For this review, take the finished solid that the model builds, in its own axes (mm). A direction names the side the tool comes from. Give positions to 0.01 mm unless a question says otherwise; leave off trailing zeros. Loops run counter-clockwise (first coordinate to the right, second up) from the corner with the lowest first, then second, coordinate; pieces in that order, holes last. Notation, with made-up numbers: (30.5, 56.5) -> (75.5, 56.5) arc R18 cw to (75.5, 73.5) -> close; hole circle Ø7 at (36, -4.5). An arc over 180 degrees is marked (long way). Answer as CSV lines item,"result". Start each with the question number.
Item 1: Add section A-A on z = -1. State the section outline as (x, y) points, plus the area to 3 significant figures.
Item 2: Clearance check with flat-ended pins moving along their axes: P1, Ø1.5, axis at y = -41.5, z = -13.5, coming from the +X side; P2, Ø5, axis at x = 1, y = -51, coming from the -Z side; P3, Ø2, axis at x = 6, y = -49.5, coming from the +Z side. State where each tip first meets the part, or that it passes through.
Item 3: Add section D-D on x = 6. State the section outline as (y, z) points, plus the area to 3 significant figures.
Item 4: Machinability: for faces 4 (the face through (5, -46, -7.498)), 5 (the face through (5.009, -45.969, -37.974)), which of the approach directions +Z, -Z, +X, -X, +Y, -Y give a long, thin tool a straight path to every point of the face, cutting with its end or side? Answer none if there is none.
Item 5: Add section B-B on y = -44. State the section outline as (x, z) points, plus the area to 3 significant figures.
Item 6: For L1, parallel to Y at x = 7.25, z = 2.5; L2, parallel to Z at x = 6.25, y = -53; L3, parallel to Z at x = 5, y = -50, list the stretches that pass through material, from the lowest coordinate up. Write a range as from..to.
Item 7: The part is to be moulded in two halves that separate along Y. For faces 1 (the face through (5.01, -42.74, 18.52)), 2 (the face through (10.16, -42, 12)), 3 (the face through (5, -30.394, -4)), say which applies: +Y half, -Y half, draft (parallel to the pull), parting line (faces both ways), or undercut.
Item 8: Add section C-C on y = -52. State the section outline as (x, z) points, plus the area to 3 significant figures.
```python
from build123d import *

# Parameters (mm, degrees)
SKETCH1_R           = 12.7
SKETCH1_R_2         = 4.28498
BOSS_EXTRUDE1_DEPTH = 10.159999949
SKETCH2_W           = 25.4
SKETCH2_H           = 16.03502
CUT_EXTRUDE1_DEPTH  = 73.464875935
FILLET1_R           = 4.28498


with BuildPart() as part:
    # Sketch1 → Boss-Extrude1 (new body)
    with BuildSketch(Plane.YZ):
        with BuildLine():
            Line((-60.873619371, 15.361912765), (-60.873619371, -22.738087235))
            ThreePointArc((-60.873619371, -22.738087235), (-45.633619371, -37.978087235), (-30.393619371, -22.738087235))
            Line((-30.393619371, -22.738087235), (-30.393619371, 15.361912765))
            ThreePointArc((-30.393619371, 15.361912765), (-45.633619371, 30.601912765), (-60.873619371, 15.361912765))
        make_face()
        with Locations(Location((-45.633619371, -22.738087235, 0), (0, 0, 270))):
            Circle(SKETCH1_R, mode=Mode.SUBTRACT)
        with Locations(Location((-45.633619371, 15.361912765, 0), (0, 0, 270))):
            Circle(SKETCH1_R_2, mode=Mode.SUBTRACT)
    extrude(amount=BOSS_EXTRUDE1_DEPTH)

    # Sketch2 → Cut-Extrude1 (cut, through all)
    with BuildSketch(Plane.YZ.offset(10.159999949)):
        with Locations((-45.633619371, 0.519422765)):
            Rectangle(SKETCH2_W, SKETCH2_H)
    extrude(amount=-CUT_EXTRUDE1_DEPTH, mode=Mode.SUBTRACT)

    # Fillet1
    fillet1_edges = [part.edges().sort_by_distance(p)[0] for p in [
        (5.079999975, -58.333619371, -7.498087235),
        (5.079999975, -58.333619371, 8.536932765),
        (5.079999975, -32.933619371, 8.536932765),
        (5.079999975, -32.933619371, -7.498087235),
    ]]
    fillet(fillet1_edges, radius=FILLET1_R)


solid = part.part
```
Computed values:
1,outline,"(0, -60.87) -> (10.16, -60.87) -> (10.16, -58.33) -> (0, -58.33) -> close; (0, -32.93) -> (10.16, -32.93) -> (10.16, -30.39) -> (0, -30.39) -> close"
1,area,"51.6 mm²"
2,P1,"through"
2,P2,"z = -37.71"
2,P3,"z = 30.33"
3,outline,"(-60.87, -22.74) arc R15.24 ccw to (-30.39, -22.74) -> (-30.39, 15.36) arc R15.24 ccw to (-60.87, 15.36) -> close; hole circle Ø25.4 at (-45.63, -22.74); hole (-58.33, -3.21) arc R4.28 ccw to (-54.05, -7.5) -> (-37.22, -7.5) arc R4.28 ccw to (-32.93, -3.21) -> (-32.93, 4.25) arc R4.28 ccw to (-37.22, 8.54) -> (-54.05, 8.54) arc R4.28 ccw to (-58.33, 4.25) -> close; hole circle Ø8.57 at (-45.63, 15.36)"
3,area,"935 mm²"
4,face 4,"+X, -X"
4,face 5,"-Z, +X, -X"
5,outline,"(0, -37.89) -> (10.16, -37.89) -> (10.16, -35.33) -> (0, -35.33) -> close; (0, -10.14) -> (10.16, -10.14) -> (10.16, -7.5) -> (0, -7.5) -> close; (0, 8.54) -> (10.16, 8.54) -> (10.16, 11.4) -> (0, 11.4) -> close; (0, 19.32) -> (10.16, 19.32) -> (10.16, 30.51) -> (0, 30.51) -> close"
5,area,"196 mm²"
6,L1,"-60.87..-58.33, -32.93..-30.39"
6,L2,"-36.08..-33.08, -12.39..-7.5, 8.54..28.7"
6,L3,"-37.34..-34.66, -10.81..-7.5, 8.54..29.96"
7,face 1,"undercut"
7,face 2,"draft"
7,face 3,"+Y half"
8,outline,"(0, -36.58) -> (10.16, -36.58) -> (10.16, -33.73) -> (0, -33.73) -> close; (0, -11.75) -> (10.16, -11.75) -> (10.16, -7.5) -> (0, -7.5) -> close; (0, 8.54) -> (10.16, 8.54) -> (10.16, 29.21) -> (0, 29.21) -> close"
8,area,"282 mm²"
